Can you work these out from the model? Positions are in its coordinate system, mm. Face numbers are marked on the shaded views. Give positions to 0.01 mm unless a question says otherwise; leave off trailing zeros. Loops run counter-clockwise (first coordinate to the right, second up) from the corner with the lowest first, then second, coordinate; pieces in that order, holes last. Notation, with made-up numbers: (-27, 53.5) -> (26, 53.5) arc R9 ccw to (26, 57.5) -> close; hole circle Ø9 at (58.25, 72.5). An arc over 180 degrees is marked (long way). Return JSON: item names as keys, results as strings. Group by question number.
Q1. Suppose I cut it at B-B, the plane y = 11.25. Please give me the cut outline in (x, z), and give its area (3 significant figures).
Q2. Thinking about a two-plate mould opening in Z: for the marked faces 1, 2, 3 and 4, which applies, pulls with the +Z half, pulls with the -Z half, needs draft (parallel to the pull), parting line crosses it, or undercut?
Q3. Will these pins go through, and if not, where does the flat tip stop? pin 1 (1.5 mm diameter, centred on x = -0.5, y = 2, fed in from +Z); pin 2 (4.5 mm diameter, centred on x = 0, z = 0, fed in from -Y); pin 3 (1.5 mm diameter, centred on x = 0, y = 5, fed in from +Z); pin 4 (1.2 mm diameter, centred on x = 0, z = 0, fed in from +Y).
Q4. I need wall thicknesses on line 1 along Z through (x, y) = (0, -3.1); line 2 along Z through (x, y) = (-0.5, 6.25); line 3 along X through (y, z) = (-4.5, 2.25). Which ranges of each line are inside material? Lowest first, please. Write a range as [from, to].
Q5. Suppose I cut it at A-A, the plane y = 2.75. Please give me the cut outline in (x, z).
```python
from build123d import *

# Parameters (mm, degrees)
FILLET2_R = 2
FILLET3_R = 1
FILLET4_R = 1


with BuildPart() as part:
    # Sketch2 → Revolve1 (revolve)
    with BuildSketch(Plane.XY, mode=Mode.PRIVATE) as revolve1_sk:
        Polygon((-1.55, 12.982183952), (-2.230367431, 0), (-5.05, 0), (-5.05, -6), (-3.95, -6), (-3.95, -1), (-0.75, -1), (-0.75, 13), align=None)
    revolve(revolve1_sk.sketch.rotate(Axis((0, -1000, 0), (0, 1, 0)), 180), axis=Axis((0, -1000, 0), (0, 1, 0)))

    # Fillet2
    fillet2_edges = [part.edges().sort_by_distance(p)[0] for p in [
        (-2.230367431, 0, 0),
    ]]
    fillet(fillet2_edges, radius=FILLET2_R)

    # Fillet3
    fillet3_edges = [part.edges().sort_by_distance(p)[0] for p in [
        (-5.05, 0, 0),
    ]]
    fillet(fillet3_edges, radius=FILLET3_R)

    # Fillet4
    # the kernel refuses this fillet: 1 mm, written as the material it takes off along each edge
    with BuildSketch(Plane(origin=(0, 12.982183952, 0), x_dir=(1, 0, 0), z_dir=(0, 0, 1))) as fillet4_piece_1:
        with BuildLine():
            CenterArc((0.599504848, -0.970794699), FILLET4_R, 3, 78.344377595)
            Line((0.75, 0.017816048), (0.753009903, 0.037588263))
            ThreePointArc((0.753009903, 0.037588263), (1.150445291, 0.028903066), (1.550445291, 0.019995042))
            Line((1.550445291, 0.019995042), (1.569972591, 0.001046719))
            Line((1.569972591, 0.001046719), (1.618106974, -0.917412024))
            Line((1.618106974, -0.917412024), (1.598134383, -0.918458743))
        make_face()
    revolve(axis=Axis((0, 12.982183952, 0), (0, 1, 0)), mode=Mode.SUBTRACT)


solid = part.part
```
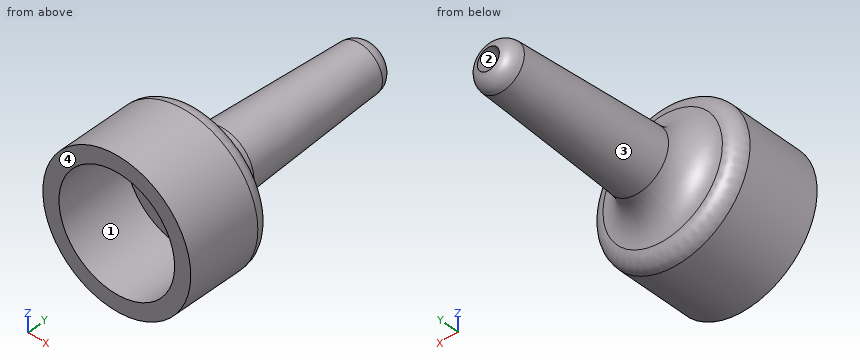
Ans:
{
 "1": {"outline": "circle Ø3.28 at (0, 0); hole circle Ø1.5 at (0, 0)", "area": "6.69 mm^2"},
 "2": {"face 1": "undercut", "face 2": "undercut", "face 3": "parting line crosses it", "face 4": "needs draft"},
 "3": {"pin 1": "stops at z = 2.24", "pin 2": "stops at y = -1", "pin 3": "stops at z = 2.01", "pin 4": "passes through"},
 "4": {"line 1": "z = [-5.05, -3.95], [3.95, 5.05]", "line 2": "z = [-1.84, -0.56], [0.56, 1.84]", "line 3": "x = [-4.52, -3.25], [3.25, 4.52]"},
 "5": {"outline": "circle Ø4.17 at (0, 0); hole circle Ø1.5 at (0, 0)"}
}
